from build123d import *

# Parameters (mm, degrees)
SKETCH_1_R               = 47.5
SKETCH_1_R_2             = 33
EXTRUDE_1_DEPTH          = 5
SKETCH_2_W               = 10
SKETCH_2_H               = 20
CUT_EXTRUDE_1_DEPTH      = 25
SKETCH_3_R               = 2
CUT_EXTRUDE_2_DEPTH      = 25
PATTERN_CIRCULAR_1_COUNT = 3


with BuildPart() as part:
    # Эскиз1 → Бобышка-Вытянуть1 (new body)
    with BuildSketch(Plane(origin=(0, 0, 0), x_dir=(1, 0, 0), z_dir=(0, 1, 0))):
        with Locations(Location((0, 0, 0), (0, 0, 270))):
            Circle(SKETCH_1_R)
        with Locations(Location((0, 0, 0), (0, 0, 270))):
            Circle(SKETCH_1_R_2, mode=Mode.SUBTRACT)
    extrude(amount=EXTRUDE_1_DEPTH)

    # Эскиз2 → Вырез-Вытянуть1 (cut, symmetric)
    with BuildSketch(Plane.XY):
        with Locations((-50, 5)):
            Rectangle(SKETCH_2_W, SKETCH_2_H)
        with Locations((50, 5)):
            Rectangle(SKETCH_2_W, SKETCH_2_H)
    extrude(amount=CUT_EXTRUDE_1_DEPTH, both=True, mode=Mode.SUBTRACT)

    # Эскиз3 → Вырез-Вытянуть2 (cut, symmetric)
    with BuildSketch(Plane(origin=(0, 0, 0), x_dir=(1, 0, 0), z_dir=(0, 1, 0))):
        with Locations(Location((0, 40, 0), (0, 0, 270))):
            Circle(SKETCH_3_R)
        with Locations(Location((0, -40, 0), (0, 0, 270))):
            Circle(SKETCH_3_R)
    cut_extrude_2 = extrude(amount=CUT_EXTRUDE_2_DEPTH, both=True, mode=Mode.SUBTRACT)

    # Круговой массив1: Вырез-Вытянуть2 ×3 about axis
    pattern_circular_1_axis = Axis((0, 0, 0), (0, 1, 0))
    for i in range(1, PATTERN_CIRCULAR_1_COUNT):
        add(cut_extrude_2.rotate(pattern_circular_1_axis, i * 360 / PATTERN_CIRCULAR_1_COUNT), mode=Mode.SUBTRACT)


solid = part.part
Work out the finished part from the listing and answer in its coordinate system (mm). Coordinates: 2 decimals unless noted, no trailing zeros. Write each loop counter-clockwise with the first axis right and the second up, starting at its lowest first coordinate (ties: lowest second). Pieces come first, ordered by that corner, then holes. Notation, with made-up numbers: M 74,73.5 L 94,73.5 A18 cw 94,91.5 Z; hole C 81,-4.5 d6. An arc over 180 degrees is marked long. Answer as CSV lines item,"result". Start each with the question number.
Item 1: Flat-ended cylindrical pins translate along their axes: P1, Ø3, axis at x = -19.5, y = 0.5, coming from the -Z side; P2, Ø1, axis at y = 2.5, z = 27.5, coming from the +X side; P3, Ø1, axis at x = -9, y = 3.5, coming from the +Z side; P4, Ø3, axis at x = 0, z = -40, coming from the +Y side. Find the tip coordinate at first contact, or state that the pin passes through.
Item 2: Determine the mould class of faces 1 (the face through (-0.828, 2.465, 47.493)), 2 (the face through (-9, 5, -32)), 3 (the face through (45, 2, 0)), 4 (the face through (32.689, 2.465, 19.566)) for opening direction X: released by +X, released by -X, zero draft, split by the parting line, or undercut.
Item 3: Section C-C on y = 2.2 is taken. Write down the section's boundary in (x, z), and give its area (3 significant figures).
Item 4: Section A-A on z = 0 is taken. Write down the section's boundary in (x, y).
Item 5: Section B-B on x = -12 is taken. Write down the section's boundary in (y, z).
Item 6: Section D-D on z = -36 is taken. Write down the section's boundary in (x, y), and give its area (3 significant figures).
Item 7: Consider L1, parallel to X at y = 3.4, z = -20; L2, parallel to Z at x = 17, y = 2.6; L3, parallel to Z at x = -6, y = 2.25. Determine where each line is inside the solid, lowest interval first.
Checks:
1,P1,"stops at z = -43.96"
1,P2,"stops at x = 39.08"
1,P3,"stops at z = 46.73"
1,P4,"passes through"
2,face 1,"split by the parting line"
2,face 2,"zero draft"
2,face 3,"released by +X"
2,face 4,"undercut"
3,outline,"M -45,-15.21 A47.5 ccw 45,-15.21 L 45,15.21 A47.5 ccw -45,15.21 Z; hole C -34.64,-20 d4; hole C -34.64,20 d4; hole C 0,0 d66; hole C 0,-40 d4; hole C 0,40 d4; hole C 34.64,-20 d4; hole C 34.64,20 d4"
3,area,"3,490 mm²"
4,outline,"M -45,0 L -33,0 L -33,5 L -45,5 Z; M 33,0 L 45,0 L 45,5 L 33,5 Z"
5,outline,"M 0,-45.96 L 5,-45.96 L 5,-30.74 L 0,-30.74 Z; M 0,30.74 L 5,30.74 L 5,45.96 L 0,45.96 Z"
6,outline,"M -30.99,0 L 30.99,0 L 30.99,5 L -30.99,5 Z"
6,area,"310 mm²"
7,L1,"x = -43.08 to -36.64, -32.64 to -26.25, 26.25 to 32.64, 36.64 to 43.08"
7,L2,"z = -44.35 to -28.28, 28.28 to 44.35"
7,L3,"z = -47.12 to -32.45, 32.45 to 47.12"
